Work out the finished part from the listing and answer in its coordinate system (mm). A direction names the side the tool comes from. Round coordinates to 2 decimals unless told otherwise and drop trailing zeros. Write each loop counter-clockwise with the first axis right and the second up, starting at its lowest first coordinate (ties: lowest second). Pieces come first, ordered by that corner, then holes.
1. Find section B-B (x = 0). Write down the section's boundary in (y, z), and give its area (3 significant figures).
2. Find section A-A (y = 5.08). Write down the section's boundary in (x, z) (3 decimals).
3. Find section D-D (z = -4.75). Write down the section's boundary in (x, y), and give its area (3 significant figures).
4. A tool of negligible diameter and unlimited length cuts with its end or side. For faces 1 (the face through (-10, 10.16, 0)), 2 (the face through (10, 10.16, 0)), 3 (the face through (5, 0, -1)), 4 (the face through (0, 10.16, -8)), 5 (the face through (-5.12, 1.98, -0.69)), from which of +Z, -Z, +X, -X, +Y, -Y can it reach the whole face along a straight path? Write none if from no direction.
5. Flat-ended cylindrical pins translate along their axes: pin 1 Ø1.5 at (x, z) = (8, -4.5) entering from +Y; pin 2 Ø5 at (y, z) = (3.5, 1.5) entering from -X; pin 3 Ø4 at (x, z) = (9.5, 5) entering from -Y; pin 4 Ø5 at (x, y) = (9, 39) entering from -Z. Find the tip coordinate at first contact, or state that the pin passes through.
6. Straight lines are drawn through the part: probe 1 along X at (y, z) = (3, 6.5); probe 2 along X at (y, z) = (11, 0); probe 3 along Y at (x, z) = (6.4, 0) (1 decimal). For each, find the intervals that lie inside material, in ascending order.
7. Find section C-C (z = 2). Write down the section's boundary in (x, y).
8. Determine the mould class of faces 6 (the face through (-3.815, 19.948, -12.114)), 7 (the face through (-7.62, 2.75, 2.4)), 8 (the face through (-2.52, 16.6, 0.33)) for opening direction X: pulls with the +X half, pulls with the -X half, needs draft (parallel to the pull), parting line crosses it, or undercut.
```python
from build123d import *

# Parameters (mm, degrees)
CUT_EXTRUDE1_DEPTH = 10.16
SKETCH3_R          = 3.175
CUT_EXTRUDE2_DEPTH = 52.61889964
FILLET1_R          = 2.54


with BuildPart() as part:
    # Sketch1 → Revolve1 (revolve)
    with BuildSketch(Plane.XY, mode=Mode.PRIVATE) as revolve1_sk:
        with BuildLine():
            Line((0, 0), (0, 5.602635041))
            Line((0, 5.602635041), (-2.54, 5.602635041))
            Line((-2.54, 5.602635041), (-2.54, 22.86))
            ThreePointArc((-2.54, 22.86), (-10.394222266, 34.299587235), (0, 43.492688289))
            Line((0, 43.492688289), (0, 45.72))
            ThreePointArc((0, 45.72), (-8.980256121, 42.000256121), (-12.7, 33.02))
            Line((-12.7, 33.02), (-12.7, 0))
            Line((-12.7, 0), (0, 0))
        make_face()
    revolve(revolve1_sk.sketch.rotate(Axis((0, 0, 0), (0, 1, 0)), 270), axis=Axis((0, 0, 0), (0, 1, 0)))

    # Sketch2 → Cut-Extrude1 (cut)
    with BuildSketch(Plane.XZ):
        with BuildLine():
            Line((-2.54, 12.443407893), (-2.54, -12.443407893))
            ThreePointArc((-2.54, -12.443407893), (0, -12.7), (2.54, -12.443407893))
            Line((2.54, -12.443407893), (2.54, 12.443407893))
            ThreePointArc((2.54, 12.443407893), (0, 12.7), (-2.54, 12.443407893))
        make_face()
        with BuildLine():
            Line((-7.62, 10.16), (-7.62, -10.16))
            ThreePointArc((-7.62, -10.16), (-12.7, 0), (-7.62, 10.16))
        make_face()
        with BuildLine():
            Line((7.62, 10.16), (7.62, -10.16))
            ThreePointArc((7.62, -10.16), (12.7, 0), (7.62, 10.16))
        make_face()
    extrude(amount=-CUT_EXTRUDE1_DEPTH, mode=Mode.SUBTRACT)

    # Sketch3 → Cut-Extrude2 (cut, through all)
    with BuildSketch(Plane.ZY.offset(7.62)):
        with Locations((0, 5.08)):
            Circle(SKETCH3_R)
    extrude(amount=-CUT_EXTRUDE2_DEPTH, mode=Mode.SUBTRACT)

    # Fillet1
    fillet1_edges = [part.edges().sort_by_distance(p)[0] for p in [
        (5.206715654, 0, 11.583613948),
        (-5.206715654, 0, 11.583613948),
    ]]
    fillet(fillet1_edges, radius=FILLET1_R)


solid = part.part
```
Worked answers:
1. outline: (10.16, -12.7) - (33.02, -12.7) arc R12.7 ccw to (33.02, 12.7) - (10.16, 12.7) - (10.16, 2.54) - (22.86, 2.54) arc R10.47 cw (long way) to (22.86, -2.54) - (10.16, -2.54) - close
1. area: 426 mm2
2. outline: (-7.62, -10.16) arc R12.7 ccw to (-2.54, -12.443) - (-2.54, -3.175) - (-7.62, -3.175) - close; (-7.62, 3.175) - (-2.54, 3.175) - (-2.54, 12.443) arc R12.7 ccw to (-7.62, 10.16) - close; (2.54, -12.443) arc R12.7 ccw to (7.62, -10.16) - (7.62, -3.175) - (2.54, -3.175) - close; (2.54, 3.175) - (7.62, 3.175) - (7.62, 10.16) arc R12.7 ccw to (2.54, 12.443) - close
3. outline: (-11.78, 10.16) - (-7.62, 10.16) - (-7.62, 0) - (-2.54, 0) - (-2.54, 10.16) - (2.54, 10.16) - (2.54, 0) - (7.62, 0) - (7.62, 10.16) - (11.78, 10.16) - (11.78, 33.02) arc R11.78 ccw to (-11.78, 33.02) - close; hole circle Ø18.67 at (0, 33.02)
3. area: 586 mm2
4. face 1: +Z, -Z, -X, -Y
4. face 2: +Z, -Z, +X, -Y
4. face 3: +Z, -Z, +X, -X, -Y
4. face 4: +Z, -Z, -Y
4. face 5: +X, -X
5. pin 1: stops at y = 42.52
5. pin 2: stops at x = -7.62
5. pin 3: stops at y = 0
5. pin 4: stops at z = -9.61
6. probe 1: x = -7.62 to -2.54, 2.54 to 7.62
6. probe 2: x = -12.7 to -2.54, 2.54 to 12.7
6. probe 3: y = 0 to 1.9, 8.3 to 24.7, 41.3 to 44
7. outline: (-12.54, 10.16) - (-7.62, 10.16) - (-7.62, 7.55) - (-2.54, 7.55) - (-2.54, 10.16) - (-1.57, 10.16) - (-1.57, 22.86) arc R10.28 cw (long way) to (1.57, 22.86) - (1.57, 10.16) - (2.54, 10.16) - (2.54, 7.55) - (7.62, 7.55) - (7.62, 10.16) - (12.54, 10.16) - (12.54, 33.02) arc R12.54 ccw to (-12.54, 33.02) - close; (-7.62, 0) - (-2.54, 0) - (-2.54, 2.61) - (-7.62, 2.61) - close; (2.54, 0) - (7.62, 0) - (7.62, 2.61) - (2.54, 2.61) - close
8. face 6: parting line crosses it
8. face 7: pulls with the -X half
8. face 8: undercut
